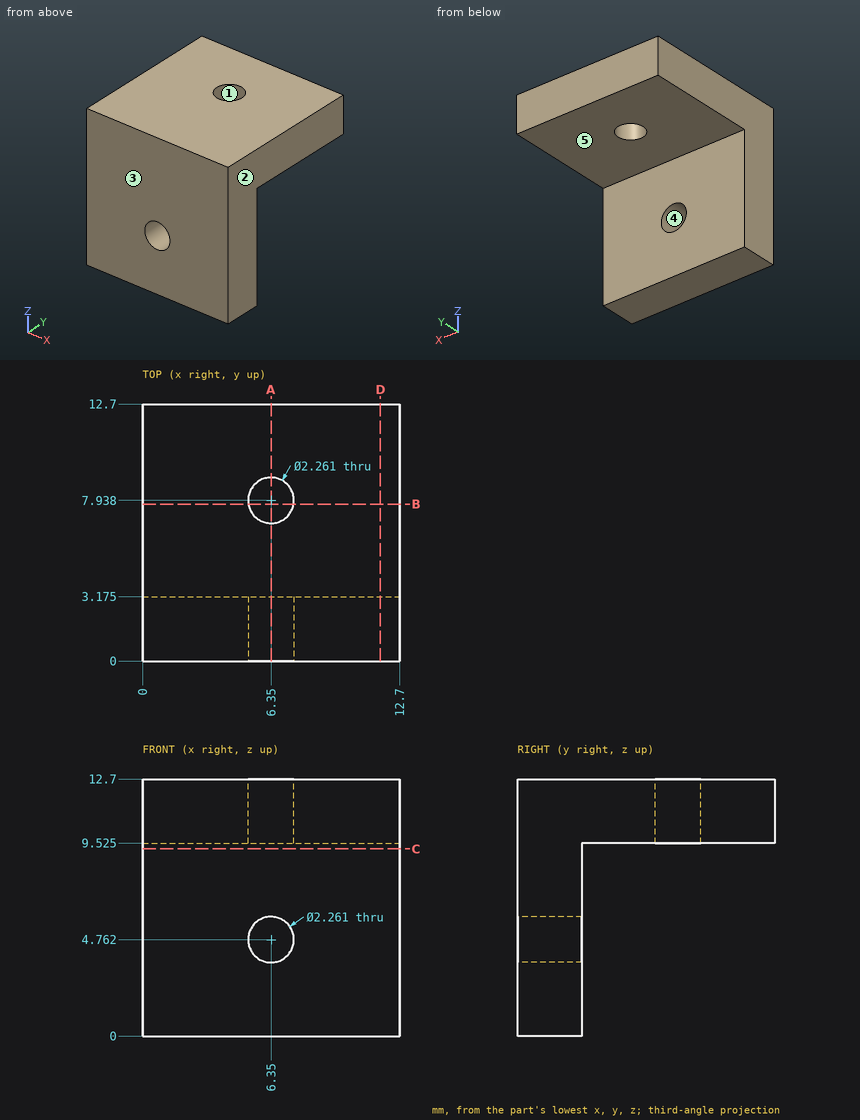
Job drawing, mm, ordinate dimensions from the low corner. One solid piece. A direction names the side the tool comes from. Round coordinates to 2 decimals unless told otherwise and drop trailing zeros. Loops run counter-clockwise (first coordinate to the right, second up) from the corner with the lowest first, then second, coordinate; pieces in that order, holes last.
(1) Wall check: line 1 along Y through (x, z) = (6.35, 10.45); line 2 along Z through (x, y) = (6.35, 1.25); line 3 along Y through (x, z) = (4, 3) (1 decimal). Give the ranges that are in metal, low to high.
(2) Cut at B-B (y = 7.75). Give the cut face in (x, z) (1 decimal).
(3) Drop flat-ended pins along their axis: pin 1 (1.4 mm diameter, centred on x = 6.35, y = 7.94, fed in from -Z); pin 2 (1.5 mm diameter, centred on x = 8.5, z = 7, fed in from +Y) (1 decimal); pin 3 (5 mm diameter, centred on x = 9, y = 8, fed in from -Z) (1 decimal). Give the stop position or say it passes through.
(4) Cut at A-A (x = 6.35). Give the cut face in (y, z) (1 decimal).
(5) Cut at C-C (z = 9.25). Give the cut face in (x, y) (1 decimal).
(6) Two-plate mould, pull along Y, no slides. Class the marked faces 1, 2 and 3: +Y half, -Y half, draft (parallel to the pull), parting line (faces both ways), or undercut.
(7) Which spindle directions (+Z, -Z, +X, -X, +Y, -Y) get a long thin tool onto all of the face, cutting with end or side? Do the marked faces 4 and 5. Say none if no direction does.
(8) Cut at D-D (x = 11.75). Give the cut face in (y, z) (1 decimal).
Findings below:
1. line 1: y = 0 to 6.81, 9.07 to 12.7
1. line 2: z = 0 to 3.63, 5.89 to 12.7
1. line 3: y = 0 to 3.2
2. outline: (0, 9.5) - (5.2, 9.5) - (5.2, 12.7) - (0, 12.7) - close; (7.5, 9.5) - (12.7, 9.5) - (12.7, 12.7) - (7.5, 12.7) - close
3. pin 1: passes through
3. pin 2: stops at y = 3.2
3. pin 3: stops at z = 9.5
4. outline: (0, 0) - (3.2, 0) - (3.2, 3.6) - (0, 3.6) - close; (0, 5.9) - (3.2, 5.9) - (3.2, 9.5) - (6.8, 9.5) - (6.8, 12.7) - (0, 12.7) - close; (9.1, 9.5) - (12.7, 9.5) - (12.7, 12.7) - (9.1, 12.7) - close
5. outline: (0, 0) - (12.7, 0) - (12.7, 3.2) - (0, 3.2) - close
6. face 1: undercut
6. face 2: draft
6. face 3: -Y half
7. face 4: +Y, -Y
7. face 5: -Z, +X, -X, +Y
8. outline: (0, 0) - (3.2, 0) - (3.2, 9.5) - (12.7, 9.5) - (12.7, 12.7) - (0, 12.7) - close
